Can you work these out from the model? Positions are in its coordinate system, mm. Face numbers are marked on the shaded views. A direction names the side the tool comes from. Give positions to 0.01 mm unless a question says otherwise; leave off trailing zeros. Write each loop counter-clockwise with the first axis right and the second up, starting at its lowest first coordinate (ties: lowest second). Pieces come first, ordered by that corner, then holes. Notation, with made-up numbers: (22.25, 67.25) -> (59.25, 67.25) arc R27 cw to (59.25, 89.25) -> close; hole circle Ø5 at (-11, -33.5). An arc over 180 degrees is marked (long way). One line per item, written item: value.
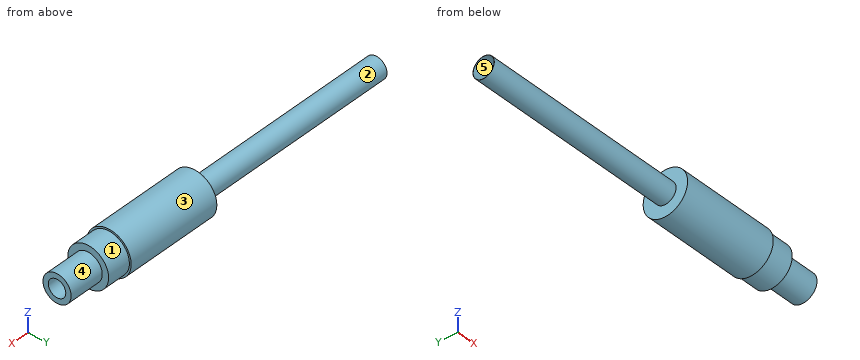
Autodesk Inventor part; units mm, degrees
ref_plane "Work Plane1" through (0, 0, 1.6) normal (0, 0, 1) x (1, 0, 0)
ref_plane "Work Plane2" through (15, 0, 0) normal (1, 0, 0) x (0, 1, 0)
ref_plane "XZ Plane" through (0, 0, 0) normal (0, 1, 0) x (-1, 0, 0)
sketch "Sketch2" plane through (0, 0, 0) normal (0, 1, 0) x (-1, 0, 0)
  line L0 (0, 0) -> (-5, 0)
  line L1 (-5, 0) -> (-10, 1.6)
  line L2 (-10, 1.6) -> (-15, 1.6)
  dimension "d0" = 1.6
  dimension "d1" = 5
  dimension "d2" = 5
  dimension "d3" = 5
sketch "Sketch3" plane through (0, 0, 0) normal (1, 0, 0) x (0, 1, 0)
  circle A0 centre (0, 0) radius 0.9
  dimension "d4" = 1.8
sweep "Sweep1" [suppressed]
ref_plane "Work Plane1" through (0, 0, 1.6) normal (0, 0, 1) x (1, 0, 0)
sketch "Sketch4" plane through (0, 0, 1.6) normal (0, 0, 1) x (1, 0, 0)
  line L0 (25, -15) -> (25, -66.3933)
  line L1 (0, 0) -> (10, 0)
  arc A0 (25, -15) -> (10, 0) centre (10, -15) ccw
  dimension "d33" = 15
  dimension "d34" = 25
  dimension "d35" = 51.3933
ref_plane "Work Plane2" through (15, 0, 0) normal (1, 0, 0) x (0, 1, 0)
sketch "Sketch5" plane through (15, 0, 0) normal (1, 0, 0) x (0, 1, 0)
  circle A0 centre (0, 1.6) radius 0.9
  point P0 (0, 0)
  dimension "d16" = 1.6
  dimension "d17" = 1.8
sweep "Sweep2" [suppressed]
sketch "Sketch7" plane through (0, 0, 0) normal (1, 0, 0) x (0, 1, 0)
  circle A0 centre (0, 0) radius 0.75
  circle A1 centre (0, 0) radius 1.2065
  dimension "d21" = 2.413
  dimension "d36" = 1.5
extrude "Extrusion1" add sketch "Sketch7" against normal blind 3.048
sketch "Sketch8" plane through (-3.048, 0, 0) normal (-1, 0, 0) x (0, 0, 1)
  circle A0 centre (0, 0) radius 0.9
  circle A1 centre (0, 0) radius 1.2065
  circle A2 centre (0, 0) radius 1.7526
  dimension "d24" = 3.5052
extrude "Extrusion2" add sketch "Sketch8" along normal blind 2.032 contours A1 | A2
sketch "Sketch9" plane through (-5.08, 0, 0) normal (-1, 0, 0) x (0, 0, 1)
  circle A0 centre (0, 0) radius 0.9
  circle A1 centre (0, 0) radius 1.7526
  circle A2 centre (0, 0) radius 1.905
  dimension "d27" = 3.81
extrude "Extrusion3" add sketch "Sketch9" along normal blind 8.382 contours A1 | A2
sketch "Sketch10" plane through (-13.462, 0, 0) normal (-1, 0, 0) x (0, 0, 1)
  circle A0 centre (0, 0) radius 0.9
  circle A1 centre (0, 0) radius 1.905
  circle A2 centre (0, 0) radius 0.9144
  dimension "d30" = 1.8288
extrude "Extr_RG-178_72mils" add sketch "Sketch10" along normal blind 17.78 contours A2
properties part number "mmcx_coax_tip"
1) If we section it at D-D (x = -8): Write out the boundary of the cut face in (y, z) (3 decimals).
Answer list:
outline: circle Ø3.81 at (0, 0); hole circle Ø1.8 at (0, 0)
2) We'd pull the mould along Z, two halves only. Please class the marked faces 4 and 5: released by +Z, released by -Z, zero draft, split by the parting line, or undercut.
Answer list:
face 4: split by the parting line
face 5: undercut
3) I need wall thicknesses on L1, parallel to Z at x = -1.45, y = 0; L2, parallel to Y at x = -9, z = 0 (3 decimals); L3, parallel to X at y = -1.05, z = -0.95. Which ranges of each line are inside material? Lowest first, please.
Answer list:
L1: z = -1.21 to -0.75, 0.75 to 1.21
L2: y = -1.905 to -0.9, 0.9 to 1.905
L3: x = -13.46 to -3.05
4) Will these pins go through, and if not, where does the flat tip stop? pin 1 (1.5 mm diameter, centred on x = -22, y = -1.5, fed in from -Z); pin 2 (1 mm diameter, centred on x = -25, y = 0.5, fed in from +Z); pin 3 (1.4 mm diameter, centred on y = 0, z = 0, fed in from -X); pin 4 (1.5 mm diameter, centred on x = -17, z = -1, fed in from -Y).
Answer list:
pin 1: stops at z = -0.52
pin 2: stops at z = 0.91
pin 3: passes through
pin 4: stops at y = -0.88
5) If we section it at C-C (x = -27.5): Write out the boundary of the cut face in (y, z), and give its area (3 significant figures).
Answer list:
outline: circle Ø1.83 at (0, 0); hole circle Ø1.8 at (0, 0)
area: 0.0821 mm^2
6) For the marked faces 1, 2 and 3, which set-ups out of +Z, -Z, +X, -X, +Y, -Y let a thin tool reach every point of the face, with its end or its side?
Answer list:
face 1: +X
face 2: -X
face 3: +X, -X
